Can you work these out from the model? Positions are in its coordinate system, mm. A direction names the side the tool comes from. Coordinates: 2 decimals unless noted, no trailing zeros. Order: outer loops, then holes, each group sorted by start corner. A loop starts at its lowest first (then second) coordinate and runs counter-clockwise, first axis right, second up. Notation, with made-up numbers: (11, 57) -> (40, 57) arc R14 ccw to (40, 65) -> close; hole circle Ø8 at (10.25, 40.5). An arc over 180 degrees is marked (long way). Write item = value, one per line.
```python
from build123d import *

# Parameters (mm, degrees)
F1_DEPTH = 19.05


with BuildPart() as f1:
    # F0 (on Front) → F1 (new body)
    with BuildSketch(Plane.XZ):
        with BuildLine():
            ThreePointArc((-32.870578, 0), (-1.120578, 31.75), (30.629422, 0))
            Line((30.629422, 0), (30.629422, -152.4))
            Line((30.629422, -152.4), (43.329422, 0))
            ThreePointArc((43.329422, 0), (-1.120578, 44.45), (-45.570578, 0))
            Line((-45.570578, 0), (-32.870578, -152.4))
            Line((-32.870578, -152.4), (-32.870578, 0))
        make_face()
    extrude(amount=F1_DEPTH)


solid = f1.part
```
Item 1: I want a section at A-A, the plane z = -15. Please give me the cut outline in (x, y).
A:
outline = (-44.32, -19.05) -> (-32.87, -19.05) -> (-32.87, 0) -> (-44.32, 0) -> close; (30.63, -19.05) -> (42.08, -19.05) -> (42.08, 0) -> (30.63, 0) -> close
Item 2: For faces 1 (the flat face through (30.629, -9, -75)), 2 (the flat face through (36.89, -9.39, -77.27)), which set-ups out of +Z, -Z, +X, -X, +Y, -Y let a thin tool reach every point of the face, with its end or its side?
A:
face_1 = -Z, +Y, -Y
face_2 = -Z, +X, +Y, -Y
Item 3: I want a section at D-D, the plane x = -3. Please give me the cut outline in (y, z), plus the area to 3 significant figures.
A:
outline = (-19.05, 31.69) -> (0, 31.69) -> (0, 44.41) -> (-19.05, 44.41) -> close
area = 242 mm2
Item 4: If I drill on probe 1 along X at (y, z) = (-11.75, 1); probe 2 along X at (y, z) = (-11.25, 25.5); probe 3 along Z at (x, y) = (-23, -8.75), over which ranges is the centre line in solid material (lowest first)?
A:
probe_1 = -45.56 to -32.85, 30.61 to 43.32
probe_2 = -37.53 to -20.04, 17.8 to 35.29
probe_3 = 23.01 to 38.69
Item 5: I want a section at C-C, the plane z = -120. Please give me the cut outline in (x, y).
A:
outline = (-35.57, -19.05) -> (-32.87, -19.05) -> (-32.87, 0) -> (-35.57, 0) -> close; (30.63, -19.05) -> (33.33, -19.05) -> (33.33, 0) -> (30.63, 0) -> close
Item 6: I want a section at B-B, the plane y = -17. Please give me the cut outline in (x, z), plus the area to 3 significant figures.
A:
outline = (-45.57, 0) -> (-32.87, -152.4) -> (-32.87, 0) arc R31.75 cw to (30.63, 0) -> (30.63, -152.4) -> (43.33, 0) arc R44.45 ccw to start
area = 3,460 mm2
Item 7: I'm going to push flat-ended pins straight in: P1, Ø3, axis at x = -12.5, y = -16, coming from the -Z side; P2, Ø8, axis at y = -16.5, z = -45, coming from the +X side; P3, Ø5.5, axis at y = -6.5, z = -46, coming from the -X side; P4, Ø4, axis at x = -35, z = -110, coming from the +Y side. Where does each tip first touch, or does it pass through?
A:
P1 = 29.02
P2 = 39.91
P3 = -41.97
P4 = 0
Item 8: If we mould it in two halves opening along X, with no side actions, what happens to faces 3 (the flat face through (-32.871, -9, -77)), 4 (the cylindrical face through (-0.14, -9.39, 44.44)), 5 (the flat face through (32, 0, -17))? For each: pulls with the +X half, pulls with the -X half, needs draft (parallel to the pull), parting line crosses it, or undercut.
A:
face_3 = undercut
face_4 = parting line crosses it
face_5 = needs draft
